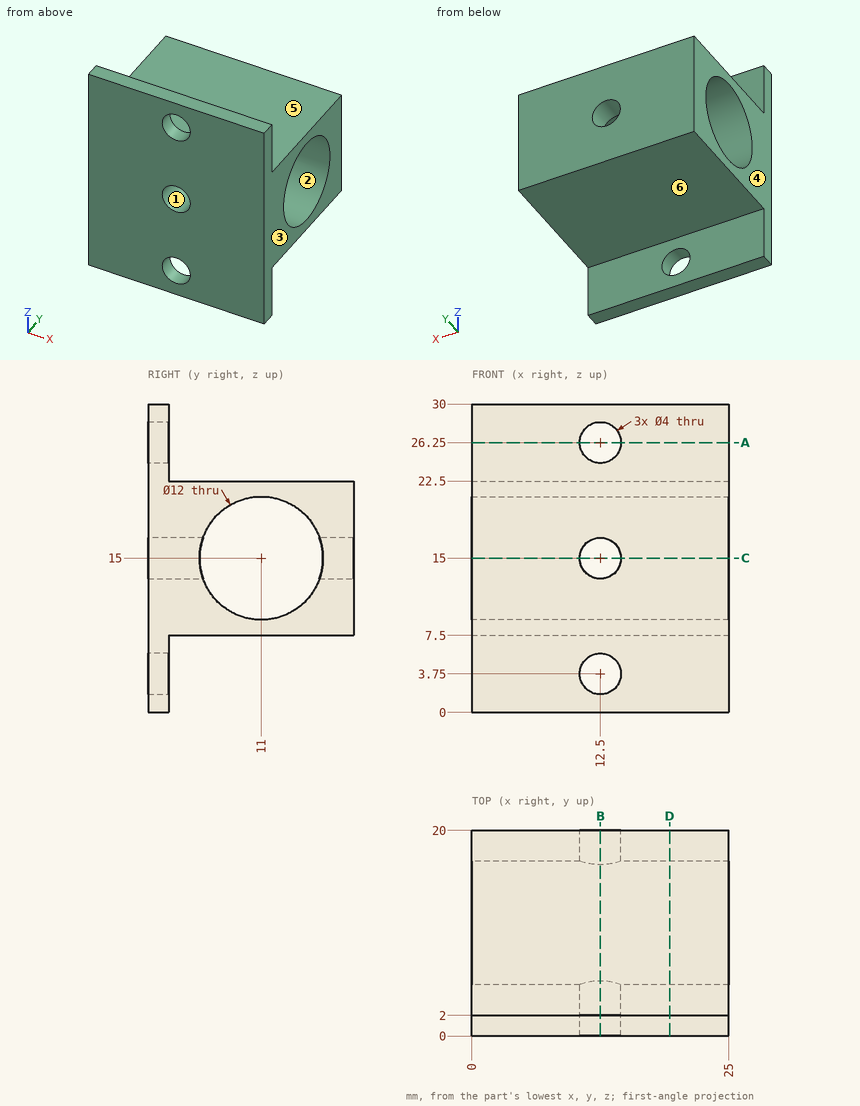
Source: three-view drawing plus pictorial views. Frame: mm from the lowest corner of the part. A direction names the side the tool comes from. Round coordinates to 2 decimals unless told otherwise and drop trailing zeros. Order: outer loops, then holes, each group sorted by start corner. A loop starts at its lowest first (then second) coordinate and runs counter-clockwise, first axis right, second up. Notation, with made-up numbers: M -27.5,77 L -3.5,77 A26 cw -3.5,104 Z; hole C 49.5,87.25 d7. An arc over 180 degrees is marked long. One line per item, written item: value.
(1) Pin query (flat end, axial travel): P1, Ø2, axis at x = 7.5, z = 26.5, coming from the +Y side; P2, Ø4.5, axis at x = 12.5, z = 26.25, coming from the -Y side; P3, Ø9, axis at x = 8, y = 13.5, coming from the +Z side. Return the tip coordinate at first contact, or that it passes through.
Result sheet:
P1: y = 2
P2: y = 0
P3: z = 22.5
(2) Pull-direction query (X, two-part tool) for the marked faces 1, 2 and 3; classes: pulls with the +X half, pulls with the -X half, needs draft (parallel to the pull), parting line crosses it, or undercut.
Result sheet:
face 1: undercut
face 2: needs draft
face 3: pulls with the +X half
(3) Cut plane B-B (x = 12.5). Return the cut outline in (y, z).
Result sheet:
outline: M 0,0 L 2,0 L 2,1.75 L 0,1.75 Z; M 0,5.75 L 2,5.75 L 2,7.5 L 20,7.5 L 20,13 L 16.66,13 A6 cw 5.34,13 L 0,13 Z; M 0,17 L 5.34,17 A6 cw 16.66,17 L 20,17 L 20,22.5 L 2,22.5 L 2,24.25 L 0,24.25 Z; M 0,28.25 L 2,28.25 L 2,30 L 0,30 Z
(4) Cut plane C-C (z = 15). Return the cut outline in (x, y), and give its area (3 significant figures).
Result sheet:
outline: M 0,0 L 10.5,0 L 10.5,5 L 0,5 Z; M 0,17 L 10.5,17 L 10.5,20 L 0,20 Z; M 14.5,0 L 25,0 L 25,5 L 14.5,5 Z; M 14.5,17 L 25,17 L 25,20 L 14.5,20 Z
area: 168 mm2
(5) Line query: probe 1 along X at (y, z) = (1.95, 15); probe 2 along Y at (x, z) = (9.75, 15); probe 3 along Z at (x, y) = (10.25, 11.25). Output: solid intervals per line, ascending. Write a range as [from, to].
Result sheet:
probe 1: [0, 10.5], [14.5, 25]
probe 2: [0, 5], [17, 20]
probe 3: [7.5, 9.01], [20.99, 22.5]
(6) Reachability of the marked faces 4, 5 and 6 from +Z, -Z, +X, -X, +Y, -Y: full face, straight path, thin tool, end or side. Return the list, or none.
Result sheet:
face 4: +Z, -Z, -X, +Y, -Y
face 5: +Z, +X, -X, +Y
face 6: -Z, +X, -X, +Y
(7) Cut plane D-D (x = 19.25). Return the cut outline in (y, z).
Result sheet:
outline: M 0,0 L 2,0 L 2,7.5 L 20,7.5 L 20,22.5 L 2,22.5 L 2,30 L 0,30 Z; hole C 11,15 d12
(8) Cut plane A-A (z = 26.25). Return the cut outline in (x, y).
Result sheet:
outline: M 0,0 L 10.5,0 L 10.5,2 L 0,2 Z; M 14.5,0 L 25,0 L 25,2 L 14.5,2 Z
